The figure shows three views and two pictorial views of one solid part (mm, origin at its lowest corner). Answer the questions. A direction names the side the tool comes from. Give positions to 0.01 mm unless a question says otherwise; leave off trailing zeros. Loops run counter-clockwise (first coordinate to the right, second up) from the corner with the lowest first, then second, coordinate; pieces in that order, holes last. Notation, with made-up numbers: (61, -29.75) - (73, -29.75) arc R23 ccw to (73, -2.75) - close; hole circle Ø2 at (33.25, 20). An arc over 180 degrees is marked (long way). Write each question's results on one line, items separated by ' | '.
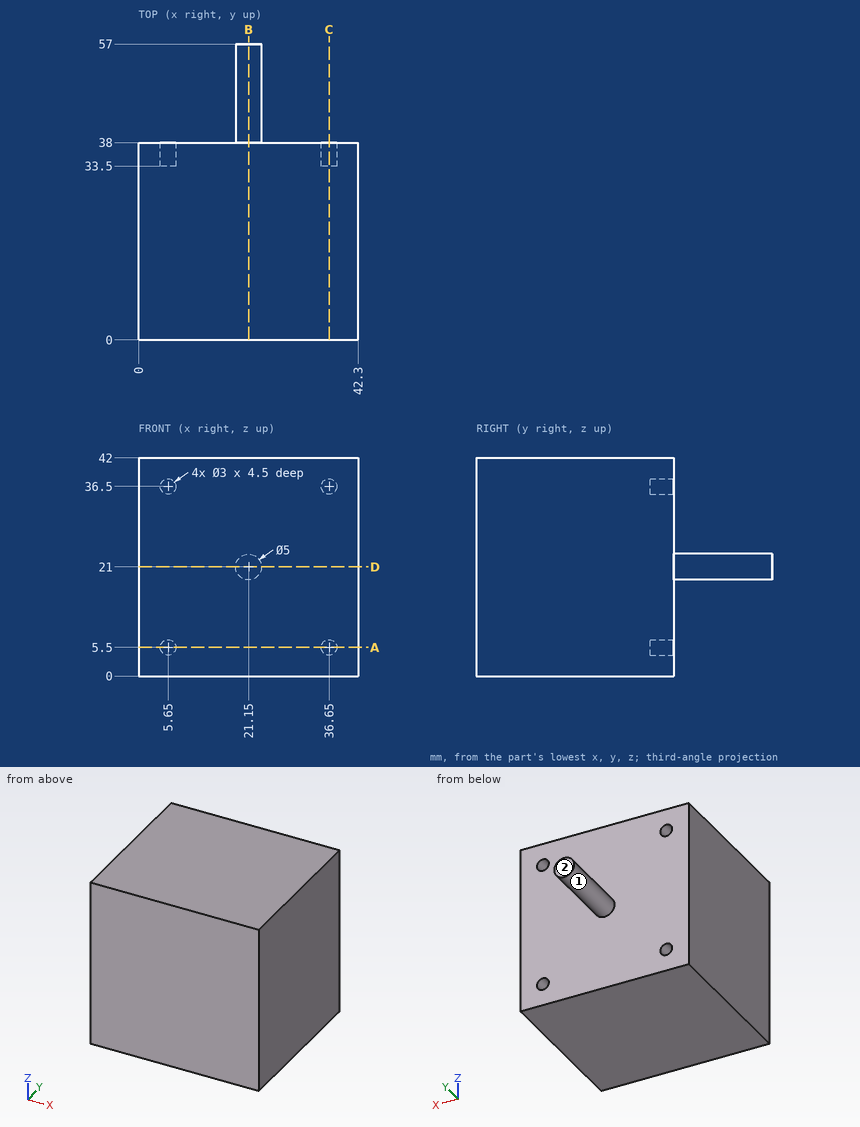
Item 1: A cutting plane is placed at C-C, the plane x = 36.65. Determine the outline of the cut face in (y, z), plus the area to 3 significant figures.
Values found:
outline: (0, 0) - (38, 0) - (38, 4) - (33.5, 4) - (33.5, 7) - (38, 7) - (38, 35) - (33.5, 35) - (33.5, 38) - (38, 38) - (38, 42) - (0, 42) - close | area: 1,570 mm²
Item 2: A cutting plane is placed at B-B, the plane x = 21.15. Determine the outline of the cut face in (y, z).
Values found:
outline: (0, 0) - (38, 0) - (38, 18.5) - (57, 18.5) - (57, 23.5) - (38, 23.5) - (38, 42) - (0, 42) - close
Item 3: For the marked faces 1 and 2, determine the directions among +Z, -Z, +X, -X, +Y, -Y from which every point of the face is accessible in a straight line to the end or side of a thin tool.
Values found:
face 1: +Y | face 2: +Z, -Z, +X, -X, +Y
Item 4: Find the intervals of material crossed by line 1 along Z through (x, y) = (36.65, 36.95); line 2 along X through (y, z) = (36.05, 5.5); line 3 along Z through (x, y) = (36, 37), in increasing order. Write a range as [from, to].
Values found:
line 1: z = [0, 4], [7, 35], [38, 42] | line 2: x = [0, 4.15], [7.15, 35.15], [38.15, 42.3] | line 3: z = [0, 4.15], [6.85, 35.15], [37.85, 42]
Item 5: Flat-ended cylindrical pins translate along their axes: P1, Ø3, axis at y = 46, z = 20.5, coming from the -X side; P2, Ø2.5, axis at x = 5.65, z = 5.5, coming from the +Y side; P3, Ø10, axis at x = 6, y = 6.5, coming from the -Z side; P4, Ø3.5, axis at x = 6, z = 36, coming from the +Y side. Find the tip coordinate at first contact, or state that the pin passes through.
Values found:
P1: stops at x = 18.65 | P2: stops at y = 33.5 | P3: stops at z = 0 | P4: stops at y = 38
Item 6: A cutting plane is placed at D-D, the plane z = 21. Determine the outline of the cut face in (x, y), plus the area to 3 significant figures.
Values found:
outline: (0, 0) - (42.3, 0) - (42.3, 38) - (23.65, 38) - (23.65, 57) - (18.65, 57) - (18.65, 38) - (0, 38) - close | area: 1,700 mm²
Item 7: A cutting plane is placed at A-A, the plane z = 5.5. Determine the outline of the cut face in (x, y), plus the area to 3 significant figures.
Values found:
outline: (0, 0) - (42.3, 0) - (42.3, 38) - (38.15, 38) - (38.15, 33.5) - (35.15, 33.5) - (35.15, 38) - (7.15, 38) - (7.15, 33.5) - (4.15, 33.5) - (4.15, 38) - (0, 38) - close | area: 1,580 mm²
